Here's the drawing with two shaded views (mm, measured from the low corner). I have some questions. A direction names the side the tool comes from. Give positions to 0.01 mm unless a question says otherwise; leave off trailing zeros. Write each loop counter-clockwise with the first axis right and the second up, starting at its lowest first coordinate (ties: lowest second). Pieces come first, ordered by that corner, then holes. Notation, with made-up numbers: (12.25, 28.5) -> (36.25, 28.5) arc R18 ccw to (36.25, 61.5) -> close; hole circle Ø11 at (78.5, -35.5). An arc over 180 degrees is marked (long way). Put each result on its own line as item: value. Start each with the question number.
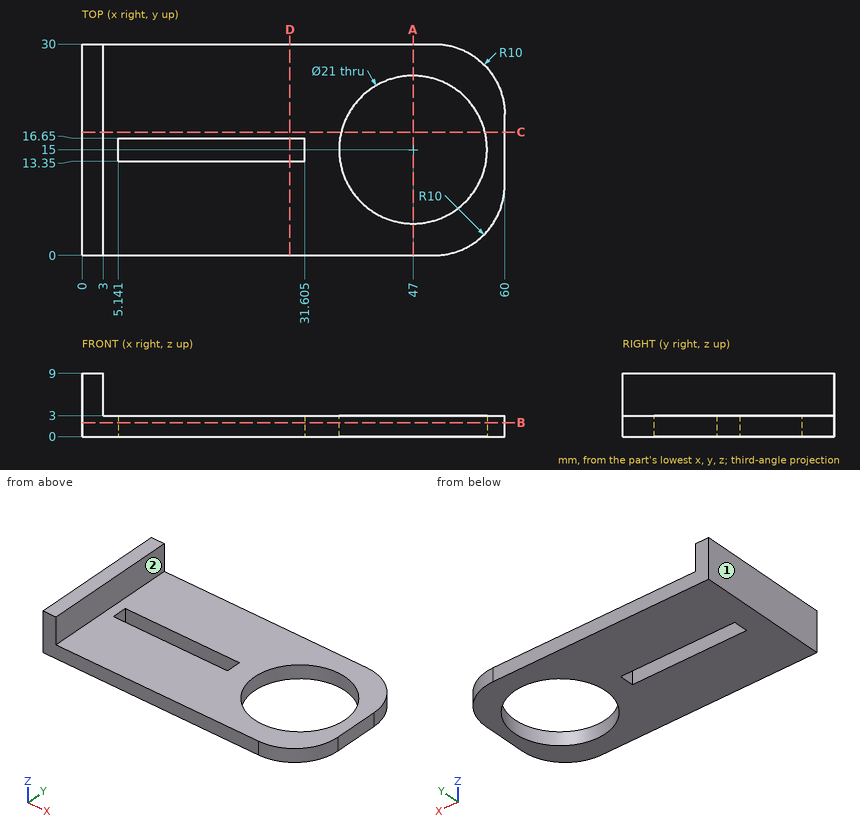
1) I want a section at B-B, the plane z = 2. Write out the boundary of the cut face in (x, y) (3 decimals).
2) I need wall thicknesses on probe 1 along Y at (x, z) = (47, 1.95); probe 2 along Y at (x, z) = (30, 2.75); probe 3 along X at (y, z) = (24, 4.25). Which ranges of each line are inside material? Lowest first, please.
3) Which directions (+Z, -Z, +X, -X, +Y, -Y) give clear straight access to the entire face, cutting with the end or side of a thin tool? Please do the marked faces 1 and 2.
4) I want a section at D-D, the plane x = 29.5. Write out the boundary of the cut face in (y, z), and give its area (3 significant figures).
5) I want a section at C-C, the plane y = 17.5. Write out the boundary of the cut face in (x, z), and give its area (3 significant figures).
6) I'm going to push flat-ended pins straight in: pin 1 Ø1 at (x, z) = (31.5, 4.5) entering from +Y; pin 2 Ø10 at (x, y) = (47, 9) entering from +Z; pin 3 Ø5 at (y, z) = (14.5, 6) entering from +X. Where does each tip first touch, or does it pass through?
7) I want a section at A-A, the plane x = 47. Write out the boundary of the cut face in (y, z).
Established:
1. outline: (0, 0) -> (50, 0) arc R10 ccw to (60, 10) -> (60, 20) arc R10 ccw to (50, 30) -> (0, 30) -> close; hole (5.141, 13.35) -> (31.605, 13.35) -> (31.605, 16.65) -> (5.141, 16.65) -> close; hole circle Ø21 at (47, 15)
2. probe 1: y = 0 to 4.5, 25.5 to 30
2. probe 2: y = 0 to 13.35, 16.65 to 30
2. probe 3: x = 0 to 3
3. face 1: +Z, -Z, -X, +Y, -Y
3. face 2: +Z, +X, +Y, -Y
4. outline: (0, 0) -> (13.35, 0) -> (13.35, 3) -> (0, 3) -> close; (16.65, 0) -> (30, 0) -> (30, 3) -> (16.65, 3) -> close
4. area: 80.1 mm2
5. outline: (0, 0) -> (36.8, 0) -> (36.8, 3) -> (3, 3) -> (3, 9) -> (0, 9) -> close; (57.2, 0) -> (60, 0) -> (60, 3) -> (57.2, 3) -> close
5. area: 137 mm2
6. pin 1: passes through
6. pin 2: stops at z = 3
6. pin 3: stops at x = 3
7. outline: (0, 0) -> (4.5, 0) -> (4.5, 3) -> (0, 3) -> close; (25.5, 0) -> (30, 0) -> (30, 3) -> (25.5, 3) -> close
